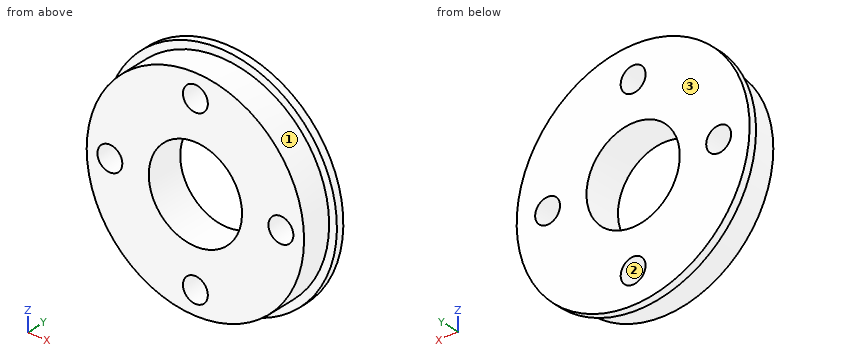
from build123d import *

# Parameters (mm, degrees)
SKETCH_1_R               = 13.98
EXTRUDE_1_DEPTH          = 4
SKETCH_2_R               = 14.98
EXTRUDE_2_DEPTH          = 1
SKETCH_3_R               = 7.97
EXTRUDE_3_DEPTH          = 2
SKETCH_5_R               = 6
SKETCH_5_R_2             = 1.6
CUT_EXTRUDE_1_DEPTH      = 21
SKETCH_7_R               = 13.98
SKETCH_7_R_2             = 7.97
CUT_EXTRUDE_4_DEPTH      = 0.1
CUT_EXTRUDE_5_DEPTH      = 10
CUT_EXTRUDE_5_DEPTH_BACK = 10
SKETCH_8_W               = 15.94
SKETCH_8_H               = 2.1


with BuildPart() as part:
    # Sketch 1 → Extrude 1 (new body)
    with BuildSketch(Plane(origin=(0, 0, 0), x_dir=(1, 0, 0), z_dir=(0, 1, 0))):
        with Locations(Location((0, 0, 0), (0, 0, 270))):
            Circle(SKETCH_1_R)
    extrude(amount=EXTRUDE_1_DEPTH)

    # Sketch 2 → Extrude 2 (add)
    with BuildSketch(Plane(origin=(0, 4, 0), x_dir=(1, 0, 0), z_dir=(0, 1, 0))):
        with Locations(Location((0, 0, 0), (0, 0, 270))):
            Circle(SKETCH_2_R)
    extrude(amount=EXTRUDE_2_DEPTH)

    # Sketch 3 → Extrude 3 (add)
    with BuildSketch(Plane.XZ):
        with Locations(Location((0, 0, 0), (0, 0, 270))):
            Circle(SKETCH_3_R)
    extrude(amount=EXTRUDE_3_DEPTH)

    # Sketch 5 → Cut-Extrude 1 (cut)
    with BuildSketch(Plane.XZ.offset(2)):
        with Locations(Location((0, 0, 0), (0, 0, 270))):
            Circle(SKETCH_5_R)
        with Locations(Location((0, 11, 0), (0, 0, 90))):
            Circle(SKETCH_5_R_2)
        with Locations(Location((11, 0, 0), (0, 0, 90))):
            Circle(SKETCH_5_R_2)
        with Locations(Location((0, -11, 0), (0, 0, 90))):
            Circle(SKETCH_5_R_2)
        with Locations(Location((-11, 0, 0), (0, 0, 90))):
            Circle(SKETCH_5_R_2)
    extrude(amount=-CUT_EXTRUDE_1_DEPTH, mode=Mode.SUBTRACT)

    # Sketch 7 → Cut-Extrude 4 (cut)
    with BuildSketch(Plane.XZ):
        with Locations(Location((0, 0, 0), (0, 0, 270))):
            Circle(SKETCH_7_R)
        with Locations(Location((0, 0, 0), (0, 0, 270))):
            Circle(SKETCH_7_R_2, mode=Mode.SUBTRACT)
    extrude(amount=-CUT_EXTRUDE_4_DEPTH, mode=Mode.SUBTRACT)

    # Sketch 8 → Cut-Extrude 5 (cut, two sides: drawn at the far end of the back side and taken through both)
    with BuildSketch(Plane(origin=(0, 0, 0), x_dir=(0, 0, -1), z_dir=(1, 0, 0)).offset(-CUT_EXTRUDE_5_DEPTH_BACK)):
        with Locations((0, -0.95)):
            Rectangle(SKETCH_8_W, SKETCH_8_H)
    extrude(amount=CUT_EXTRUDE_5_DEPTH + CUT_EXTRUDE_5_DEPTH_BACK, mode=Mode.SUBTRACT)


solid = part.part
Work out the finished part from the listing and answer in its coordinate system (mm). Face numbers are marked on the shaded views. Give positions to 0.01 mm unless a question says otherwise; leave off trailing zeros. Write each loop counter-clockwise with the first axis right and the second up, starting at its lowest first coordinate (ties: lowest second). Pieces come first, ordered by that corner, then holes. Notation, with made-up numbers: (86.25, 73) - (133.25, 73) arc R8 cw to (133.25, 87) - close; hole circle Ø7 at (-26, 23.25). An arc over 180 degrees is marked (long way). One line per item, written item: value. Start each with the question number.
1. Find section B-B (z = 0). Write down the section's boundary in (x, y), then the cut area to 3 significant figures.
2. For a pull along Z with two mould halves and no side action, classify the marked faces 1, 2 and 3 as +Z half, -Z half, draft (parallel to the pull), parting line (faces both ways), or undercut.
3. Consider probe 1 along X at (y, z) = (2.95, 0); probe 2 along Z at (x, y) = (11, 3.6); probe 3 along X at (y, z) = (0.5, -12). Determine where each line is inside the solid, lowest interval first.
4. Find section D-D (z = -11). Write down the section's boundary in (x, y), then the cut area to 3 significant figures.
5. Given pin 1 (3 mm diameter, centred on x = -11, z = 0, fed in from +Y); pin 2 (2 mm diameter, centred on y = 1, z = 5, fed in from +X), each flat-ended and moving along its own axis, determine where each tip first touches the part or whether it passes through.
6. Find section A-A (x = 0). Write down the section's boundary in (y, z), then the cut area to 3 significant figures.
7. Find section C-C (y = 1.85). Write down the section's boundary in (x, z), then the cut area to 3 significant figures.
Geometry results:
1. outline: (-14.98, 4) - (-13.98, 4) - (-13.98, 0.1) - (-12.6, 0.1) - (-12.6, 5) - (-14.98, 5) - close; (-9.4, 0.1) - (-6, 0.1) - (-6, 5) - (-9.4, 5) - close; (6, 0.1) - (9.4, 0.1) - (9.4, 5) - (6, 5) - close; (12.6, 0.1) - (13.98, 0.1) - (13.98, 4) - (14.98, 4) - (14.98, 5) - (12.6, 5) - close
1. area: 48.8 mm2
2. face 1: parting line
2. face 2: undercut
2. face 3: draft
3. probe 1: -13.98 to -12.6, -9.4 to -6, 6 to 9.4, 12.6 to 13.98
3. probe 2: -8.63 to -1.6, 1.6 to 8.63
3. probe 3: -7.17 to -1.25, 1.25 to 7.17
4. outline: (-10.17, 4) - (-8.63, 4) - (-8.63, 0.1) - (-1.6, 0.1) - (-1.6, 5) - (-10.17, 5) - close; (1.6, 0.1) - (8.63, 0.1) - (8.63, 4) - (10.17, 4) - (10.17, 5) - (1.6, 5) - close
4. area: 72.0 mm2
5. pin 1: through
5. pin 2: x = 13.4
6. outline: (0.1, -13.98) - (4, -13.98) - (4, -14.98) - (5, -14.98) - (5, -12.6) - (0.1, -12.6) - close; (0.1, -9.4) - (5, -9.4) - (5, -6) - (0.1, -6) - close; (0.1, 6) - (5, 6) - (5, 9.4) - (0.1, 9.4) - close; (0.1, 12.6) - (5, 12.6) - (5, 14.98) - (4, 14.98) - (4, 13.98) - (0.1, 13.98) - close
6. area: 48.8 mm2
7. outline: circle Ø27.96 at (0, 0); hole circle Ø3.2 at (-11, 0); hole circle Ø12 at (0, 0); hole circle Ø3.2 at (0, -11); hole circle Ø3.2 at (0, 11); hole circle Ø3.2 at (11, 0)
7. area: 469 mm2
